For this review, take the finished solid that the model builds, in its own axes (mm). A direction names the side the tool comes from. Coordinates: 2 decimals unless noted, no trailing zeros. Loops run counter-clockwise (first coordinate to the right, second up) from the corner with the lowest first, then second, coordinate; pieces in that order, holes last.
```python
from build123d import *

# Parameters (mm, degrees)
F1_DEPTH = 3


# Not quite as in the source:
# - ends of sketch curves that miss each other by under 0.0002 mm in the source are joined


with BuildPart() as f1:
    # F0 (on Front) → F1 (new body)
    with BuildSketch(Plane.XZ):
        with BuildLine():
            Line((27.6752540097, 25.9776275605), (-32.3247459903, 25.9776275605))
            ThreePointArc((-32.3247459903, 25.9776275605), (-36.2904670893, 25.5805114342), (-40.0987030081, 24.4049331771))
            Line((-40.0987030081, 24.4049331771), (-40.0987030081, 19.4049331771))
            Line((-40.0987030081, 19.4049331771), (-42.7675568515, 19.4049331771))
            Line((-42.7675568515, 19.4049331771), (-42.7675568515, 23.0348166993))
            ThreePointArc((-42.7675568515, 23.0348166993), (-49.7726143017, 15.7537152948), (-52.3247459903, 5.9776275605))
            Line((-52.3247459903, 5.9776275605), (-52.3247459903, 0.9776275605))
            ThreePointArc((-52.3247459903, 0.9776275605), (-46.4668816141, -13.1645080632), (-32.3247459903, -19.0223724395))
            Line((-32.3247459903, -19.0223724395), (-32.3247459903, -9.0223724395))
            Line((-32.3247459903, -9.0223724395), (-29.3247459903, -9.0223724395))
            Line((-29.3247459903, -9.0223724395), (-29.3247459903, -19.0223724395))
            Line((-29.3247459903, -19.0223724395), (24.6752540097, -19.0223724395))
            Line((24.6752540097, -19.0223724395), (24.6752540097, -9.0223724395))
            Line((24.6752540097, -9.0223724395), (27.6752540097, -9.0223724395))
            Line((27.6752540097, -9.0223724395), (27.6752540097, -19.0223724395))
            ThreePointArc((27.6752540097, -19.0223724395), (41.8173896334, -13.1645080632), (47.6752540097, 0.9776275605))
            Line((47.6752540097, 0.9776275605), (47.6752540097, 5.9776275605))
            ThreePointArc((47.6752540097, 5.9776275605), (46.6766261397, 12.2184493954), (43.7804682921, 17.8360453688))
            ThreePointArc((43.7804682921, 17.8360453688), (65.3177378121, 34.4466284435), (92.4979172096, 33.4449816105))
            ThreePointArc((92.4979172096, 33.4449816105), (93.2694445512, 33.2995729147), (94.0374965073, 33.4623435853))
            ThreePointArc((94.0374965073, 33.4623435853), (101.2901547391, 39.0961583347), (104.8859376265, 47.5466769297))
            ThreePointArc((104.8859376265, 47.5466769297), (110.0970401084, 56.2336783381), (104.1383245347, 64.4259484991))
            ThreePointArc((104.1383245347, 64.4259484991), (97.5285801831, 60.0432380566), (99.0521934878, 52.2602133107))
            ThreePointArc((99.0521934878, 52.2602133107), (96.8833215141, 44.3091582137), (89.9362853313, 39.8749765827))
            ThreePointArc((89.9362853313, 39.8749765827), (60.6981355661, 41.6708405362), (38.0764996773, 23.060194363))
            ThreePointArc((38.0764996773, 23.060194363), (33.0765808814, 25.2344618804), (27.6752540097, 25.9776275605))
        make_face()
    extrude(amount=F1_DEPTH)


solid = f1.part
```
Q1. For pin 1 Ø1 at (x, y) = (41, -2) entering from +Z; pin 2 Ø1 at (x, y) = (63.5, -2) entering from -Z; pin 3 Ø0.8 at (x, y) = (-41, -2) entering from +Z, all flat-tipped, find the tip position at first contact; note any pin that passes through.
Q2. Consider section C-C (x = 16). State the section outline as (y, z) points, then the cut area to 3 significant figures.
Q3. The part is to be moulded in two halves that separate along Z. For faces 1 (the face through (97.575, -1.479, 60.151)), 2 (the face through (101.21, -1.48, 38.99)), 3 (the face through (10, 0, 14)), say which applies: +Z half, -Z half, draft (parallel to the pull), parting line (faces both ways), or undercut.
Q4. Machinability: for faces 4 (the face through (96.95, -1.48, 44.4)), 5 (the face through (47.675, -1, 3)), 6 (the face through (-31, -1, -9.022)), which of the approach directions +Z, -Z, +X, -X, +Y, -Y give a long, thin tool a straight path to every point of the face, cutting with its end or side? Answer none if there is none.
Q5. Wall thickness on probe 1 along X at (y, z) = (-2, -11); probe 2 along Z at (x, y) = (10, -1.7); probe 3 along X at (y, z) = (-2, -12): over which ranges is each line inside the solid? List them lowest first.
Q6. Consider section B-B (z = -13.5). State the section outline as (x, y) points, then the cut area to 3 significant figures.
Q7. Consider section D-D (z = 3). State the section outline as (x, y) points, then the cut area to 3 significant figures.
Q8. Consider section A-A (y = -0.7). State the section outline as (x, z) points, then the cut area to 3 significant figures.
Model answer:
1. pin 1: stops at z = 28.23
1. pin 2: stops at z = 33.62
1. pin 3: stops at z = 19.4
2. outline: (-3, -19.02) - (0, -19.02) - (0, 25.98) - (-3, 25.98) - close
2. area: 135 mm2
3. face 1: undercut
3. face 2: -Z half
3. face 3: draft
4. face 4: +Y, -Y
4. face 5: -Z, +X, +Y, -Y
4. face 6: -Z, +Y, -Y
5. probe 1: x = -48.34 to -32.32, -29.32 to 24.68, 27.68 to 43.69
5. probe 2: z = -19.02 to 25.98
5. probe 3: x = -47.54 to -32.32, -29.32 to 24.68, 27.68 to 42.89
6. outline: (-46.12, -3) - (-32.32, -3) - (-32.32, 0) - (-46.12, 0) - close; (-29.32, -3) - (24.68, -3) - (24.68, 0) - (-29.32, 0) - close; (27.68, -3) - (41.47, -3) - (41.47, 0) - (27.68, 0) - close
6. area: 245 mm2
7. outline: (-52.32, -3) - (47.68, -3) - (47.68, 0) - (-52.32, 0) - close
7. area: 300 mm2
8. outline: (-52.32, 0.98) arc R20 ccw to (-32.32, -19.02) - (-32.32, -9.02) - (-29.32, -9.02) - (-29.32, -19.02) - (24.68, -19.02) - (24.68, -9.02) - (27.68, -9.02) - (27.68, -19.02) arc R20 ccw to (47.68, 0.98) - (47.68, 5.98) arc R20 ccw to (43.78, 17.84) arc R40 cw to (92.5, 33.44) arc R2 ccw to (94.04, 33.46) arc R18.27 ccw to (104.89, 47.55) arc R9.18 ccw to (104.14, 64.43) arc R7.13 ccw to (99.05, 52.26) arc R11.45 cw to (89.94, 39.87) arc R40 ccw to (38.08, 23.06) arc R20 ccw to (27.68, 25.98) - (-32.32, 25.98) arc R20 ccw to (-40.1, 24.4) - (-40.1, 19.4) - (-42.77, 19.4) - (-42.77, 23.03) arc R20 ccw to (-52.32, 5.98) - close
8. area: 4,800 mm2
